```python
from build123d import *

# Parameters (mm, degrees)
SKETCH1_W           = 60
SKETCH1_H           = 60
BOSS_EXTRUDE1_DEPTH = 350
SKETCH3_W           = 43.312374626
SKETCH3_H           = 40
CUT_EXTRUDE2_DEPTH  = 375
SKETCH4_R           = 15
CUT_EXTRUDE3_DEPTH  = 375


with BuildPart() as part:
    # Sketch1 → Boss-Extrude1 (new body)
    with BuildSketch(Plane.XY):
        Rectangle(SKETCH1_W, SKETCH1_H)
    extrude(amount=BOSS_EXTRUDE1_DEPTH)

    # Sketch3 → Cut-Extrude2 (cut)
    with BuildSketch(Plane(origin=(0, 0, 0), x_dir=(-1, 0, 0), z_dir=(0, 0, -1))):
        Rectangle(SKETCH3_W, SKETCH3_H)
    extrude(amount=-CUT_EXTRUDE2_DEPTH, mode=Mode.SUBTRACT)

    # Sketch4 → Cut-Extrude3 (cut)
    with BuildSketch(Plane(origin=(30, 0, 0), x_dir=(0, 0, -1), z_dir=(1, 0, 0))):
        with Locations((-80, 0)):
            Circle(SKETCH4_R)
    cut_extrude3 = extrude(amount=-CUT_EXTRUDE3_DEPTH, mode=Mode.SUBTRACT)

    # Mirror1: Cut-Extrude3 across plane
    add(cut_extrude3.mirror(Plane(origin=(0, 0, 175), x_dir=(1, 0, 0), z_dir=(0, 0, -1))), mode=Mode.SUBTRACT)


solid = part.part
```
Geometry check sheet. Reference: the model listing, model coordinates, mm. A direction names the side the tool comes from. Give positions to 0.01 mm unless a question says otherwise; leave off trailing zeros. Order: outer loops, then holes, each group sorted by start corner. A loop starts at its lowest first (then second) coordinate and runs counter-clockwise, first axis right, second up.
1. Section check B-B, the plane y = 0. Enter the section's corners in (x, z).
2. Section check D-D, the plane z = 135. Enter the section's corners in (x, y).
3. Gauge pin test, flat end, axial feed: pin 1 Ø24 at (y, z) = (0, 270) entering from -X. Record the tip position at first contact, or that the pin passes through.
4. Section check C-C, the plane z = 80. Enter the section's corners in (x, y).
5. Access from +Z, -Z, +X, -X, +Y, -Y to the whole of each face (thin tool, end or side, straight path). Record for faces 5 (the face through (-21.656, 0, 173)), 6 (the face through (-25.77, -5.745, 283.856)).
6. Thickness scan on L1, parallel to Y at x = 7.5, z = 65; L2, parallel to X at y = -13.5, z = 126; L3, parallel to Y at x = -27.75, z = 270. Record the ranges inside material, lowest first.
7. Section check A-A, the plane x = -12.5. Enter the section's corners in (y, z).
8. Release check for a two-part mould opening along Z. For faces 1 (the face through (-0.4, 20.4, 350)), 2 (the face through (-0.4, 20.4, 0)), 3 (the face through (25.887, -5.745, 283.856)), 4 (the face through (0, -30, 173)) record: pulls with the +Z half, pulls with the -Z half, needs draft (parallel to the pull), parting line crosses it, or undercut.
Values follow:
1. outline: (-30, 0) - (-21.66, 0) - (-21.66, 65) - (-30, 65) - close; (-30, 95) - (-21.66, 95) - (-21.66, 255) - (-30, 255) - close; (-30, 285) - (-21.66, 285) - (-21.66, 350) - (-30, 350) - close; (21.66, 0) - (30, 0) - (30, 65) - (21.66, 65) - close; (21.66, 95) - (30, 95) - (30, 255) - (21.66, 255) - close; (21.66, 285) - (30, 285) - (30, 350) - (21.66, 350) - close
2. outline: (-30, -30) - (30, -30) - (30, 30) - (-30, 30) - close; hole (-21.66, -20) - (21.66, -20) - (21.66, 20) - (-21.66, 20) - close
3. pin 1: passes through
4. outline: (-30, -30) - (30, -30) - (30, -15) - (21.66, -15) - (21.66, -20) - (-21.66, -20) - (-21.66, -15) - (-30, -15) - close; (-30, 15) - (-21.66, 15) - (-21.66, 20) - (21.66, 20) - (21.66, 15) - (30, 15) - (30, 30) - (-30, 30) - close
5. face 5: +Z, -Z
5. face 6: +X, -X
6. L1: y = -30 to -20, 20 to 30
6. L2: x = -30 to -21.66, 21.66 to 30
6. L3: y = -30 to -15, 15 to 30
7. outline: (-30, 0) - (-20, 0) - (-20, 350) - (-30, 350) - close; (20, 0) - (30, 0) - (30, 350) - (20, 350) - close
8. face 1: pulls with the +Z half
8. face 2: pulls with the -Z half
8. face 3: undercut
8. face 4: needs draft
